from build123d import *
from build123d.topology import SkipClean

# Parameters (mm, degrees)
EXTRUDE_1_DEPTH     = 13
CUT_EXTRUDE_1_DEPTH = 3
SKETCH_3_R          = 4
CUT_EXTRUDE_2_DEPTH = 2
SKETCH_4_R          = 1.65
CUT_EXTRUDE_3_DEPTH = 28.98651863
SKETCH_5_R          = 3
CUT_EXTRUDE_4_DEPTH = 1
SKETCH_6_R          = 1.65
CUT_EXTRUDE_5_DEPTH = 29.394457646
SKETCH_7_R          = 7.5
CUT_EXTRUDE_6_DEPTH = 6.3
SKETCH_8_R          = 5
CUT_EXTRUDE_7_DEPTH = 8.3
EXTRUDE_START       = 3
SKETCH_9_R          = 5
EXTRUDE_3_DEPTH     = 3


with BuildPart() as part:
    # 草图1 → 凸台-拉伸1 (new body)
    with BuildSketch(Plane(origin=(0, 0, 0), x_dir=(1, 0, 0), z_dir=(0, 1, 0))):
        with BuildLine():
            Line((-10.765, 12), (10.765, 12))
            ThreePointArc((10.765, 12), (22.765, 0), (10.765, -12))
            Line((10.765, -12), (-10.765, -12))
            ThreePointArc((-10.765, -12), (-22.765, 0), (-10.765, 12))
        make_face()
    extrude(amount=EXTRUDE_1_DEPTH)

    # 草图2 → 切除-拉伸1 (cut)
    with BuildSketch(Plane.XZ):
        Polygon((0, 12), (-1.79, 12), (-1.79, -12), (3.6, -12), (3.6, 12), align=None)
    extrude(amount=-CUT_EXTRUDE_1_DEPTH, mode=Mode.SUBTRACT)

    # 草图3 → 切除-拉伸2 (cut)
    with BuildSketch(Plane(origin=(0, 13, 0), x_dir=(1, 0, 0), z_dir=(0, 1, 0))):
        with Locations(Location((10.765, 0, 0), (0, 0, 270))):
            Circle(SKETCH_3_R)
    extrude(amount=-CUT_EXTRUDE_2_DEPTH, mode=Mode.SUBTRACT)

    # 草图4 → 切除-拉伸3 (cut, through all)
    with BuildSketch(Plane(origin=(0, 11, 0), x_dir=(1, 0, 0), z_dir=(0, 1, 0))):
        with Locations(Location((10.765, 0, 0), (0, 0, 270))):
            Circle(SKETCH_4_R)
    extrude(amount=-CUT_EXTRUDE_3_DEPTH, mode=Mode.SUBTRACT)

    # 草图5 → 切除-拉伸4 (cut)
    with BuildSketch(Plane(origin=(0, 13, 0), x_dir=(1, 0, 0), z_dir=(0, 1, 0))):
        with Locations(Location((-10.765, 0, 0), (0, 0, 270))):
            Circle(SKETCH_5_R)
    extrude(amount=-CUT_EXTRUDE_4_DEPTH, mode=Mode.SUBTRACT)

    # 草图6 → 切除-拉伸5 (cut, through all)
    with BuildSketch(Plane(origin=(0, 12, 0), x_dir=(1, 0, 0), z_dir=(0, 1, 0))):
        with Locations(Location((-10.765, 0, 0), (0, 0, 270))):
            Circle(SKETCH_6_R)
    extrude(amount=-CUT_EXTRUDE_5_DEPTH, mode=Mode.SUBTRACT)

    # 草图7 → 切除-拉伸6 (cut)
    with BuildSketch(Plane.XZ):
        with Locations(Location((10.765, 0, 0), (0, 0, 270))):
            Circle(SKETCH_7_R)
    extrude(amount=-CUT_EXTRUDE_6_DEPTH, mode=Mode.SUBTRACT)

    # 草图8 → 切除-拉伸7 (cut)
    with BuildSketch(Plane.XZ):
        with Locations(Location((-10.765, 0, 0), (0, 0, 270))):
            Circle(SKETCH_8_R)
    extrude(amount=-CUT_EXTRUDE_7_DEPTH, mode=Mode.SUBTRACT)

    # 草图9 → 凸台-拉伸3 (add)
    # profile 1 of 2: a face of its own
    with SkipClean():  # the faces are left unmerged after this step: merging them gives an invalid solid
        with BuildSketch(Plane.XZ.offset(EXTRUDE_START)):
            with BuildLine():
                Line((-10.765, -12), (-1.79, -12))
                Line((-1.79, -12), (-1.79, 12))
                Line((-1.79, 12), (-10.765, 12))
                ThreePointArc((-10.765, 12), (-22.765, 0), (-10.765, -12))
            make_face()
            with Locations(Location((-10.765, 0, 0), (0, 0, 270))):
                Circle(SKETCH_9_R, mode=Mode.SUBTRACT)
        # profile 2 of 2: a face of its own
        with BuildSketch(Plane.XZ.offset(EXTRUDE_START)):
            with BuildLine():
                Line((3.6, 12), (3.6, 2.216478062))
                ThreePointArc((3.6, 2.216478062), (18.265, 0), (3.6, -2.216478062))
                Line((3.6, -2.216478062), (3.6, -12))
                Line((3.6, -12), (10.765, -12))
                ThreePointArc((10.765, -12), (22.765, 0), (10.765, 12))
                Line((10.765, 12), (3.6, 12))
            make_face()
        extrude(amount=-EXTRUDE_3_DEPTH)


solid = part.part
Can you work these out from the model? Positions are in its coordinate system, mm. A direction names the side the tool comes from. Round coordinates to 2 decimals unless told otherwise and drop trailing zeros. Loops run counter-clockwise (first coordinate to the right, second up) from the corner with the lowest first, then second, coordinate; pieces in that order, holes last. Notation, with made-up numbers: (3, -16) - (60, -16) arc R17 ccw to (60, -2) - close; hole circle Ø1 at (54.5, 60). An arc over 180 degrees is marked (long way). Answer in a Markdown table with one row per item. Add a question column.
Q1. We'd pull the mould along X, two halves only. Please class faces 1 (the cylindrical face through (22.762, 4.888, -0.264)), 2 (the flat face through (-12, -3, -5)), 3 (the flat face through (13, 6.3, 0)): pulls with the +X half, pulls with the -X half, needs draft (parallel to the pull), parting line crosses it, or undercut.
Q2. I want a section at A-A on z = 0. Count the separate pieces of the cut face and the enclosed holes in it, and give its area (3 significant figures).
Q3. I want a section at C-C on x = 10. List the corners of the cut face in (y, z) for me.
Q4. I want a section at B-B on y = 9.75. List the corners of the cut face in (x, z) for me (3 decimals), and give its area (3 significant figures).
Q5. I want a section at D-D on x = 15.5. List the corners of the cut face in (y, z) for me.
Q6. Which directions (+Z, -Z, +X, -X, +Y, -Y) give clear straight access to the entire face, cutting with the end or side of a thin tool? Please do faces 4 (the cylindrical face through (-5.808, 2.571, 0.651)), 5 (the flat face through (-12.1, 12, 1.3)), 6 (the flat face through (3.6, 0, -7)).
Q7. I need wall thicknesses on L1, parallel to X at y = 2, z = 0 (3 decimals); L2, parallel to Z at x = 11.5, y = 3.25; L3, parallel to Y at x = -6, z = -1. Which ranges of each line are inside material? Lowest first, please.
Q8. For pin 1 Ø4.5 at (x, z) = (9.5, 1) entering from -Y; pin 2 Ø1.5 at (y, z) = (7, 4) entering from -X; pin 3 Ø3 at (x, z) = (-11.5, -1) entering from -Y; pin 4 Ø1 at (x, y) = (-0.5, 1.5) entering from +Z, each with a flat end and sliding along its axis, tell me the tip position at first contact or that it passes through.
A:
| question | item | result |
|---|---|---|
| 1 | face 1 | pulls with the +X half |
| 1 | face 2 | needs draft |
| 1 | face 3 | undercut |
| 2 | separate pieces | 3 |
| 2 | enclosed holes | 0 |
| 2 | area | 396 mm^2 |
| 3 | outline | (-3, -12) - (13, -12) - (13, -3.93) - (11, -3.93) - (11, -1.46) - (6.3, -1.46) - (6.3, -7.46) - (-3, -7.46) - close; (-3, 7.46) - (6.3, 7.46) - (6.3, 1.46) - (11, 1.46) - (11, 3.93) - (13, 3.93) - (13, 12) - (-3, 12) - close |
| 4 | outline | (-10.765, -12) - (10.765, -12) arc R12 ccw to (10.765, 12) - (-10.765, 12) arc R12 ccw to start; hole circle Ø3.3 at (-10.765, 0); hole circle Ø3.3 at (10.765, 0) |
| 4 | area | 952 mm^2 |
| 5 | outline | (-3, -11.03) - (13, -11.03) - (13, 11.03) - (-3, 11.03) - (-3, 5.82) - (6.3, 5.82) - (6.3, -5.82) - (-3, -5.82) - close |
| 6 | face 4 | -Y |
| 6 | face 5 | +Y |
| 6 | face 6 | +Z, -Z, -Y |
| 7 | L1 | -22.765 to -15.765, -5.765 to -1.79, 18.265 to 22.765 |
| 7 | L2 | -11.98 to -7.46, 7.46 to 11.98 |
| 7 | L3 | 8.3 to 13 |
| 8 | pin 1 | y = 6.3 |
| 8 | pin 2 | x = -22.32 |
| 8 | pin 3 | y = 8.3 |
| 8 | pin 4 | through |
